Source: CAD feature listing. Evaluate the final solid. Frame: model axes, mm. A direction names the side the tool comes from. Coordinates: 2 decimals unless noted, no trailing zeros. Order: outer loops, then holes, each group sorted by start corner. A loop starts at its lowest first (then second) coordinate and runs counter-clockwise, first axis right, second up.
```python
from build123d import *

# Parameters (mm, degrees)
BOSS_EXTRUDE2_DEPTH = 100
REVOLVE1_ANGLE      = 90
REVOLVE2_ANGLE      = 90
BOSS_EXTRUDE3_REACH = 1139.003
SKETCH10_W          = 80
SKETCH10_H          = 350
REVOLVE3_ANGLE      = 90
REVOLVE4_ANGLE      = 90
BOSS_EXTRUDE4_REACH = 1139.003
SKETCH14_R          = 86
SKETCH14_R_2        = 43
CUT_EXTRUDE2_DEPTH  = 135
SKETCH17_R          = 43
CUT_EXTRUDE3_DEPTH  = 583
CUT_EXTRUDE4_DEPTH  = 1340.48085047


with BuildPart() as part:
    # Sketch4 → Boss-Extrude2 (new, symmetric)
    with BuildSketch(Plane.XY):
        with BuildLine():
            Line((813.175605254, 117.699465094), (1168.175605254, 117.699465094))
            Line((1168.175605254, 117.699465094), (1168.175605254, 467.699465094))
            ThreePointArc((1168.175605254, 467.699465094), (1144.744147749, 524.268007589), (1088.175605254, 547.699465094))
            Line((1088.175605254, 547.699465094), (638.175605254, 547.699465094))
            Line((638.175605254, 547.699465094), (638.175605254, 445.457996532))
            ThreePointArc((638.175605254, 445.457996532), (691.915720625, 423.198111902), (714.175605254, 369.457996532))
            Line((714.175605254, 369.457996532), (714.175605254, 279.457996532))
            ThreePointArc((714.175605254, 279.457996532), (787.650444518, 213.251892507), (813.175605254, 117.699465094))
        make_face()
        with BuildLine():
            Line((638.175605254, 445.457996532), (638.175605254, 547.699465094))
            Line((638.175605254, 547.699465094), (188.175605254, 547.699465094))
            ThreePointArc((188.175605254, 547.699465094), (131.607062759, 524.268007589), (108.175605254, 467.699465094))
            Line((108.175605254, 467.699465094), (108.175605254, 117.699465094))
            Line((108.175605254, 117.699465094), (463.175605254, 117.699465094))
            ThreePointArc((463.175605254, 117.699465094), (488.70076599, 213.251892507), (562.175605254, 279.457996532))
            Line((562.175605254, 279.457996532), (562.175605254, 369.457996532))
            ThreePointArc((562.175605254, 369.457996532), (584.435489884, 423.198111902), (638.175605254, 445.457996532))
        make_face()
    extrude(amount=BOSS_EXTRUDE2_DEPTH, both=True)

    # Sketch7 → Revolve1 (revolve)
    with BuildSketch(Plane(origin=(0, 0, -100), x_dir=(-1, 0, 0), z_dir=(0, 0, -1))):
        with BuildLine():
            Line((-1088.175605254, 547.699465094), (-1088.175605254, 117.699465094))
            Line((-1088.175605254, 117.699465094), (-1168.175605254, 117.699465094))
            Line((-1168.175605254, 117.699465094), (-1168.175605254, 467.699465094))
            ThreePointArc((-1168.175605254, 467.699465094), (-1144.744147749, 524.268007589), (-1088.175605254, 547.699465094))
        make_face()
    revolve(axis=Axis((1088.175605254, 547.699465094, -100), (0, 1, 0)), revolution_arc=REVOLVE1_ANGLE)

    # Sketch8 → Revolve2 (revolve)
    with BuildSketch(Plane(origin=(0, 0, -100), x_dir=(-1, 0, 0), z_dir=(0, 0, -1))):
        with BuildLine():
            Line((-188.175605254, 547.699465094), (-188.175605254, 117.699465094))
            Line((-188.175605254, 117.699465094), (-108.175605254, 117.699465094))
            Line((-108.175605254, 117.699465094), (-108.175605254, 467.699465094))
            ThreePointArc((-108.175605254, 467.699465094), (-131.607062759, 524.268007589), (-188.175605254, 547.699465094))
        make_face()
    revolve(axis=Axis((188.175605254, 547.699465094, -100), (0, -1, 0)), revolution_arc=REVOLVE2_ANGLE)

    # Boss-Extrude3: up to this face of the body (flat: up to its plane)
    boss_extrude3_end = Plane(part.part.faces().sort_by_distance((188.175605254, 324.501535412, -139.079671816))[0])
    # Sketch10 → Boss-Extrude3 (add, up to the picked face)
    with BuildSketch(Plane.ZY.offset(-1088.175605254), mode=Mode.PRIVATE) as boss_extrude3_sk1:
        with BuildLine():
            Line((-100, 467.699465094), (-100, 547.699465094))
            ThreePointArc((-100, 547.699465094), (-156.568542495, 524.268007589), (-180, 467.699465094))
            Line((-180, 467.699465094), (-100, 467.699465094))
        make_face()
    boss_extrude3_tool1 = split(extrude(boss_extrude3_sk1.sketch, amount=BOSS_EXTRUDE3_REACH, mode=Mode.PRIVATE), bisect_by=boss_extrude3_end, keep=Keep.BOTH, mode=Mode.PRIVATE)
    # Sketch10 → Boss-Extrude3 (add, up to the picked face)
    with BuildSketch(Plane.ZY.offset(-1088.175605254), mode=Mode.PRIVATE) as boss_extrude3_sk2:
        with Locations((-140, 292.699465094)):
            Rectangle(SKETCH10_W, SKETCH10_H)
    boss_extrude3_tool2 = split(extrude(boss_extrude3_sk2.sketch, amount=BOSS_EXTRUDE3_REACH, mode=Mode.PRIVATE), bisect_by=boss_extrude3_end, keep=Keep.BOTH, mode=Mode.PRIVATE)
    add(boss_extrude3_tool1.solids().sort_by(Axis((1088.175605, 501.65252, -133.953055), (-1, 0, 0)))[0])
    add(boss_extrude3_tool2.solids().sort_by(Axis((1088.175605, 292.699465, -140), (-1, 0, 0)))[0])

    # Sketch11 → Revolve3 (revolve)
    with BuildSketch(Plane.XY.offset(100)):
        with BuildLine():
            Line((1088.175605254, 547.699465094), (1088.175605254, 117.699465094))
            Line((1088.175605254, 117.699465094), (1168.175605254, 117.699465094))
            Line((1168.175605254, 117.699465094), (1168.175605254, 467.699465094))
            ThreePointArc((1168.175605254, 467.699465094), (1144.744147749, 524.268007589), (1088.175605254, 547.699465094))
        make_face()
    revolve(axis=Axis((1088.175605254, 547.699465094, 100), (0, -1, 0)), revolution_arc=REVOLVE3_ANGLE)

    # Sketch12 → Revolve4 (revolve)
    with BuildSketch(Plane.XY.offset(100)):
        with BuildLine():
            Line((188.175605254, 547.699465094), (188.175605254, 117.699465094))
            Line((188.175605254, 117.699465094), (108.175605254, 117.699465094))
            Line((108.175605254, 117.699465094), (108.175605254, 467.699465094))
            ThreePointArc((108.175605254, 467.699465094), (131.607062759, 524.268007589), (188.175605254, 547.699465094))
        make_face()
    revolve(axis=Axis((188.175605254, 547.699465094, 100), (0, 1, 0)), revolution_arc=REVOLVE4_ANGLE)

    # Boss-Extrude4: up to this face of the body (flat: up to its plane)
    boss_extrude4_end = Plane(part.part.faces().sort_by_distance((1088.175605254, 324.501535412, 139.079671816))[0])
    # Sketch13 → Boss-Extrude4 (add, up to the picked face)
    with BuildSketch(Plane(origin=(188.175605254, 0, 0), x_dir=(0, 0, -1), z_dir=(1, 0, 0)), mode=Mode.PRIVATE) as boss_extrude4_sk1:
        with BuildLine():
            Line((-100, 547.699465094), (-100, 117.699465094))
            Line((-100, 117.699465094), (-180, 117.699465094))
            Line((-180, 117.699465094), (-180, 467.699465094))
            ThreePointArc((-180, 467.699465094), (-156.568542495, 524.268007589), (-100, 547.699465094))
        make_face()
    boss_extrude4_tool1 = split(extrude(boss_extrude4_sk1.sketch, amount=BOSS_EXTRUDE4_REACH, mode=Mode.PRIVATE), bisect_by=boss_extrude4_end, keep=Keep.BOTH, mode=Mode.PRIVATE)
    add(boss_extrude4_tool1.solids().sort_by(Axis((188.175605, 324.501535, 139.079672), (1, 0, 0)))[0])

    # Sketch14 → Cut-Extrude2 (cut)
    # profile 1 of 2: a face of its own
    with BuildSketch(Plane(origin=(0, 547.699465094, 0), x_dir=(1, 0, 0), z_dir=(0, 1, 0))):
        with Locations(Location((961.100411774, 0, 0), (0, 0, 270))):
            Circle(SKETCH14_R)
        with Locations(Location((961.100411774, 0, 0), (0, 0, 270))):
            Circle(SKETCH14_R_2, mode=Mode.SUBTRACT)
    # profile 2 of 2: a face of its own
    with BuildSketch(Plane(origin=(0, 547.699465094, 0), x_dir=(1, 0, 0), z_dir=(0, 1, 0))):
        with Locations(Location((315.250798734, 0, 0), (0, 0, 90))):
            Circle(SKETCH14_R)
        with Locations(Location((315.250798734, 0, 0), (0, 0, 90))):
            Circle(SKETCH14_R_2, mode=Mode.SUBTRACT)
    extrude(amount=-CUT_EXTRUDE2_DEPTH, mode=Mode.SUBTRACT)

    # Sketch17 → Cut-Extrude3 (cut)
    with BuildSketch(Plane(origin=(0, 547.699465094, 0), x_dir=(1, 0, 0), z_dir=(0, 1, 0))):
        with Locations(Location((961.100411774, 0, 0), (0, 0, 270))):
            Circle(SKETCH17_R)
        with Locations(Location((315.250798734, 0, 0), (0, 0, 270))):
            Circle(SKETCH17_R)
    extrude(amount=-CUT_EXTRUDE3_DEPTH, mode=Mode.SUBTRACT)

    # Sketch18 → Cut-Extrude4 (cut, through all)
    with BuildSketch(Plane(origin=(0, 0, -180), x_dir=(-1, 0, 0), z_dir=(0, 0, -1))):
        with BuildLine():
            Line((-714.175605254, 279.457996532), (-714.175605254, 369.457996532))
            ThreePointArc((-714.175605254, 369.457996532), (-638.175605254, 445.457996532), (-562.175605254, 369.457996532))
            Line((-562.175605254, 369.457996532), (-562.175605254, 279.457996532))
            ThreePointArc((-562.175605254, 279.457996532), (-488.70076599, 213.251892507), (-463.175605254, 117.699465094))
            Line((-463.175605254, 117.699465094), (-813.175605254, 117.699465094))
            ThreePointArc((-813.175605254, 117.699465094), (-786.461236826, 212.524069618), (-714.175605254, 279.457996532))
        make_face()
    extrude(amount=-CUT_EXTRUDE4_DEPTH, mode=Mode.SUBTRACT)


solid = part.part
```
Q1. Section query C-C on y = 433. Output: boundary loops of the cut face in (x, z).
Solutions:
outline: (108.18, -100) arc R80 ccw to (188.18, -180) - (596.48, -180) - (596.48, 180) - (188.18, 180) arc R80 ccw to (108.18, 100) - close; (679.87, -180) - (1088.18, -180) arc R80 ccw to (1168.18, -100) - (1168.18, 100) arc R80 ccw to (1088.18, 180) - (679.87, 180) - close; hole circle Ø172 at (315.25, 0); hole circle Ø172 at (961.1, 0)
Q2. Section query A-A on z = 0. Output: boundary loops of the cut face in (x, y), plus the area to 3 significant figures.
Solutions:
outline: (108.18, 117.7) - (272.25, 117.7) - (272.25, 412.7) - (229.25, 412.7) - (229.25, 547.7) - (188.18, 547.7) arc R80 ccw to (108.18, 467.7) - close; (358.25, 117.7) - (463.18, 117.7) arc R174 cw to (562.18, 279.46) - (562.18, 369.46) arc R76 cw to (714.18, 369.46) - (714.18, 279.46) arc R174 cw to (813.18, 117.7) - (918.1, 117.7) - (918.1, 412.7) - (875.1, 412.7) - (875.1, 547.7) - (401.25, 547.7) - (401.25, 412.7) - (358.25, 412.7) - close; (1004.1, 117.7) - (1168.18, 117.7) - (1168.18, 467.7) arc R80 ccw to (1088.18, 547.7) - (1047.1, 547.7) - (1047.1, 412.7) - (1004.1, 412.7) - close
area: 285,000 mm2
Q3. Pull-direction query (Z, two-part tool) for faces 4 (the cylindrical face through (130.988, 295.149, 155.943)), 5 (the cylindrical face through (489.44, 214.45, -2.52)), 6 (the cylindrical face through (1046.37, 481.14, -11.2)); classes: pulls with the +Z half, pulls with the -Z half, needs draft (parallel to the pull), parting line crosses it, or undercut.
Solutions:
face 4: pulls with the +Z half
face 5: needs draft
face 6: undercut
Q4. Pin query (flat end, axial travel): P1, Ø5, axis at y = 279, z = 113.5, coming from the +X side; P2, Ø1.5, axis at x = 905.5, z = -21, coming from the +Y side; P3, Ø12, axis at y = 488, z = -90.5, coming from the -X side. Return the tip coordinate at first contact, or that it passes through.
Solutions:
P1: stops at x = 1167.42
P2: stops at y = 412.7
P3: stops at x = 109.46
Q5. Set-up query: faces 1 (the cylindrical face through (787.186, 211.33, -140.56)), 2 (the cylindrical face through (229.983, 481.144, 11.195)), 3 (the cylindrical face through (357.885, 267.264, -5.598)). Return all of +Z, -Z, +X, -X, +Y, -Y with unobstructed straight access to the full face (end or side cutting, diameter ignored); none if empty.
Solutions:
face 1: +Z, -Z, -Y
face 2: +Y
face 3: +Y, -Y
Q6. Section query B-B on y = 193.5. Output: boundary loops of the cut face in (x, z).
Solutions:
outline: (108.18, -100) arc R80 ccw to (188.18, -180) - (478.29, -180) - (478.29, 180) - (188.18, 180) arc R80 ccw to (108.18, 100) - close; (796.6, -180) - (1088.18, -180) arc R80 ccw to (1168.18, -100) - (1168.18, 100) arc R80 ccw to (1088.18, 180) - (796.6, 180) - (796.6, 100) - (798.06, 100) - (798.06, -100) - (796.6, -100) - close; hole circle Ø86 at (315.25, 0); hole circle Ø86 at (961.1, 0)
Q7. Section query D-D on z = 129.5. Output: boundary loops of the cut face in (x, y).
Solutions:
outline: (113.81, 117.7) - (463.18, 117.7) arc R174 cw to (562.18, 279.46) - (562.18, 369.46) arc R76 cw to (714.18, 369.46) - (714.18, 279.46) arc R181.65 cw to (813.18, 117.7) - (1162.54, 117.7) - (1162.54, 467.7) arc R74.36 ccw to (1088.18, 542.06) - (188.18, 542.06) arc R74.36 ccw to (113.81, 467.7) - close
Q8. Material intervals for line 1 along X through (y, z) = (302, 0); line 2 along X through (y, z) = (471, 0); line 3 along X through (y, z) = (189, 0), sorted ascending.
Solutions:
line 1: x = 108.18 to 272.25, 358.25 to 562.18, 714.18 to 918.1, 1004.1 to 1168.18
line 2: x = 108.24 to 229.25, 401.25 to 875.1, 1047.1 to 1168.11
line 3: x = 108.18 to 272.25, 358.25 to 476.35, 800 to 918.1, 1004.1 to 1168.18
